Geometry: final body of the model. Coordinates: model frame, mm. Give positions to 0.01 mm unless a question says otherwise; leave off trailing zeros. Order: outer loops, then holes, each group sorted by start corner. A loop starts at its lowest first (then second) coordinate and runs counter-clockwise, first axis right, second up. Notation, with made-up numbers: (-19, -0.75) -> (4, -0.75) arc R16 cw to (4, 29.25) -> close; hole circle Ø7 at (-36, 65.5). An arc over 180 degrees is marked (long way). Write item = value, one per line.
```python
from build123d import *

# Parameters (mm, degrees)
PRISM003_DEPTH = 15
PRISM001_DEPTH = 3
PRISM_DEPTH    = 3
PRISM002_DEPTH = 6


with BuildPart() as prism003:
    # Prism003 → Prism003 (new body)
    with BuildSketch(Plane.XY):
        Polygon((101, 0), (-50.5, 87.468566), (-50.5, -87.468566), align=None)
    extrude(amount=PRISM003_DEPTH)


with BuildPart() as prism001:
    # Prism001 → Prism001 (new body)
    with BuildSketch(Plane.XY):
        Polygon((116, 0), (-58, 100.458947), (-58, -100.458947), align=None)
    extrude(amount=PRISM001_DEPTH)


with BuildPart() as cut:
    # Prism → Prism (new body)
    with BuildSketch(Plane.XY):
        Polygon((136, 0), (-68, 117.779455), (-68, -117.779455), align=None)
    extrude(amount=PRISM_DEPTH)

    # Cut: cut Prism001
    add(prism001.part, mode=Mode.SUBTRACT)


with BuildPart() as cut002:
    # Prism002 → Prism002 (new body)
    with BuildSketch(Plane.XY):
        Polygon((151, 0), (-75.5, 130.769836), (-75.5, -130.769836), align=None)
    extrude(amount=PRISM002_DEPTH)

    # Cut001: cut Cut
    add(cut.part, mode=Mode.SUBTRACT)

    # Cut002: cut Prism003
    add(prism003.part, mode=Mode.SUBTRACT)


solid = cut002.part
```
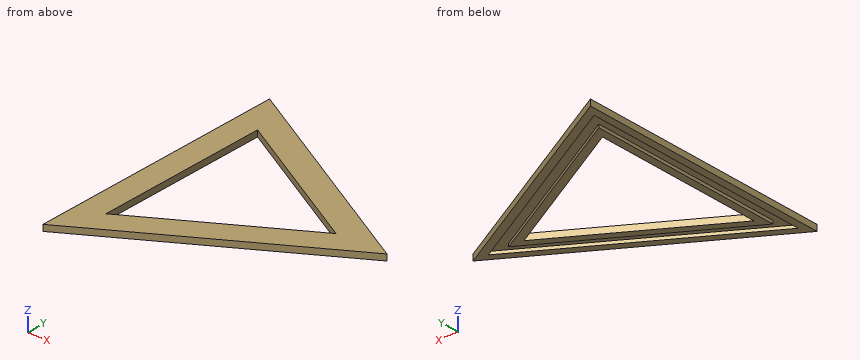
1) Section query D-D (y = 111). Output: boundary loops of the cut face in (x, z).
Check sheet entries:
outline = (-75.5, 0) -> (-68, 0) -> (-68, 3) -> (-56.26, 3) -> (-56.26, 0) -> (-41.26, 0) -> (-41.26, 6) -> (-75.5, 6) -> close
2) Section query A-A (z = 2). Output: boundary loops of the cut face in (x, y), plus the area to 3 significant figures.
Check sheet entries:
outline = (-75.5, -130.77) -> (151, 0) -> (-75.5, 130.77) -> close; (-58, -100.46) -> (116, 0) -> (-58, 100.46) -> close; hole (-68, -117.78) -> (136, 0) -> (-68, 117.78) -> close; hole (-50.5, -87.47) -> (101, 0) -> (-50.5, 87.47) -> close
area = 9,820 mm²
3) Section query C-C (x = 57). Output: boundary loops of the cut face in (y, z).
Check sheet entries:
outline = (-54.27, 0) -> (-45.61, 0) -> (-45.61, 3) -> (-34.06, 3) -> (-34.06, 0) -> (-25.4, 0) -> (-25.4, 6) -> (-54.27, 6) -> close; (25.4, 0) -> (34.06, 0) -> (34.06, 3) -> (45.61, 3) -> (45.61, 0) -> (54.27, 0) -> (54.27, 6) -> (25.4, 6) -> close
4) Section query B-B (y = -67.5). Output: boundary loops of the cut face in (x, z), plus the area to 3 significant figures.
Check sheet entries:
outline = (-75.5, 0) -> (-68, 0) -> (-68, 3) -> (-58, 3) -> (-58, 0) -> (-50.5, 0) -> (-50.5, 6) -> (-75.5, 6) -> close; (-15.91, 0) -> (-0.91, 0) -> (-0.91, 3) -> (19.09, 3) -> (19.09, 0) -> (34.09, 0) -> (34.09, 6) -> (-15.91, 6) -> close
area = 360 mm²
5) Line query: line 1 (Y direction, x = -45, z = 1.5); line 2 (Y direction, x = -46, z = 1.25); line 3 (X direction, y = 45, z = 0.5). Output: solid intervals per line, ascending. Write a range as from..to.
Check sheet entries:
line_1 = -113.16..-104.5, -92.95..-84.29, 84.29..92.95, 104.5..113.16
line_2 = -113.74..-105.08, -93.53..-84.87, 84.87..93.53, 105.08..113.74
line_3 = -75.5..-68, -58..-50.5, 23.06..38.06, 58.06..73.06
6) First-contact query: P1, Ø3, axis at y = 51.5, z = 5, coming from the +X side; P2, Ø2.5, axis at y = -52, z = 2, coming from the +X side. Flat tips, straight axial feed; report the tip coordinate or a pass-through.
Check sheet entries:
P1 = 64.4
P2 = 63.1
